from build123d import *

# Parameters (mm, degrees)
F1_DEPTH = 50.8


with BuildPart() as f1:
    # F0 (on Top) → F1 (new body)
    with BuildSketch(Plane.XY):
        with BuildLine():
            Line((58.2818202674, 67.1484221876), (-43.3181797326, 67.1484221876))
            Line((-43.3181797326, 67.1484221876), (-43.3181797326, -34.4515778124))
            Line((-43.3181797326, -34.4515778124), (58.2818202674, -34.4515778124))
            Line((58.2818202674, -34.4515778124), (58.2818202674, -13.207797377))
            ThreePointArc((58.2818202674, -13.207797377), (28.7256007029, 16.3484221876), (58.2818202674, 45.9046417521))
            Line((58.2818202674, 45.9046417521), (58.2818202674, 67.1484221876))
        make_face()
        with BuildLine():
            ThreePointArc((58.2818202674, -34.4515778124), (109.0818202674, 16.3484221876), (58.2818202674, 67.1484221876))
            Line((58.2818202674, 67.1484221876), (58.2818202674, 45.9046417521))
            ThreePointArc((58.2818202674, 45.9046417521), (79.1812235478, 37.2478254679), (87.838039832, 16.3484221876))
            ThreePointArc((87.838039832, 16.3484221876), (79.1812235478, -4.5509810928), (58.2818202674, -13.207797377))
            Line((58.2818202674, -13.207797377), (58.2818202674, -34.4515778124))
        make_face()
    extrude(amount=F1_DEPTH)


solid = f1.part
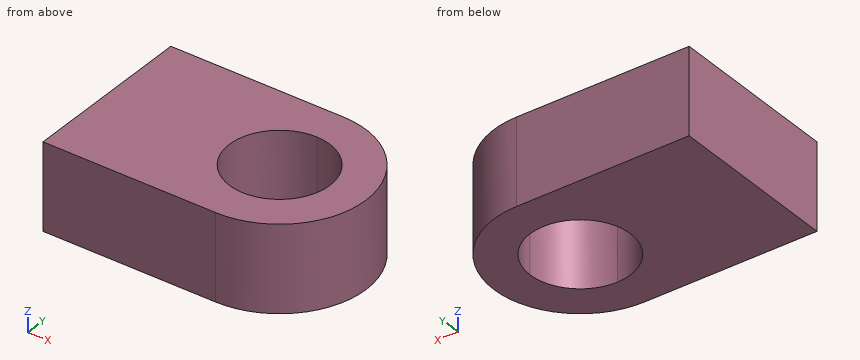
Build history of the part. All positions in model axes, mm. Coordinates: 2 decimals unless noted, no trailing zeros. Order: outer loops, then holes, each group sorted by start corner. A loop starts at its lowest first (then second) coordinate and runs counter-clockwise, first axis right, second up. Notation, with made-up numbers: M 11,63 L 59,63 A10 cw 59,79 Z; hole C 11.5,28.5 d3. An arc over 180 degrees is marked long. One line per question, with ' | ' between items. Start each with the question number.
Q1. Flat gauge pins, fed straight in: pin 1 Ø1 at (x, z) = (86.5, 29.5) entering from +Y; pin 2 Ø10 at (x, y) = (82.5, 13.5) entering from +Z; pin 3 Ø8 at (y, z) = (17.5, 16.5) entering from +X; pin 4 Ø4 at (y, z) = (49, 9) entering from +X. Where does each tip first touch, or does it go through?
Q2. Saw through at D-D (y = 49). List the corners of the cut face in (x, z), then the cut area to 3 significant figures.
Q3. Saw through at A-A (z = 30). List the corners of the cut face in (x, y).
Q4. Saw through at B-B (y = 9). List the corners of the cut face in (x, z).
Q5. Probe L1, parallel to X at y = 17, z = 23; L2, parallel to X at y = 5.5, z = 5.5; L3, parallel to Y at x = 63, z = 19.5. List the from-to ranges inside material, lowest first. Write a range as from..to.
Q6. Saw through at C-C (x = 46). List the corners of the cut face in (y, z), then the cut area to 3 significant figures.
Check values:
1) pin 1: stops at y = 58.92 | pin 2: passes through | pin 3: stops at x = 109.08 | pin 4: stops at x = 98.79
2) outline: M -43.32,0 L 97.2,0 L 97.2,50.8 L -43.32,50.8 Z | area: 7,140 mm2
3) outline: M -43.32,-34.45 L 58.28,-34.45 A50.8 ccw 58.28,67.15 L -43.32,67.15 Z; hole C 58.28,16.35 d59.11
4) outline: M -43.32,0 L 29.65,0 L 29.65,50.8 L -43.32,50.8 Z; M 86.91,0 L 108.55,0 L 108.55,50.8 L 86.91,50.8 Z
5) L1: x = -43.32..28.73, 87.83..109.08 | L2: x = -43.32..30.79, 85.78..107.91 | L3: y = -34.23..-12.83, 45.53..66.93
6) outline: M -34.45,0 L -10.54,0 L -10.54,50.8 L -34.45,50.8 Z; M 43.23,0 L 67.15,0 L 67.15,50.8 L 43.23,50.8 Z | area: 2,430 mm2
